```python
from build123d import *

# Parameters (mm, degrees)
SKETCH2_R          = 0.5
CUT_EXTRUDE1_DEPTH = 9.746515042
SKETCH3_R          = 33.25
SKETCH3_R_2        = 28.75
CUT_EXTRUDE3_DEPTH = 7.5


with BuildPart() as part:
    # Sketch1 → Revolve1 (revolve)
    with BuildSketch(Plane(origin=(0, 0, 0), x_dir=(1, 0, 0), z_dir=(0, 1, 0))):
        with BuildLine():
            Line((0, 2.406901823), (-37, 2.406901823))
            Line((-37, 2.406901823), (-37, -0.593098177))
            ThreePointArc((-37, -0.593098177), (-18.857679345, -5.739925328), (0, -5.593098177))
            Line((0, -5.593098177), (0, 2.406901823))
        make_face()
    revolve(axis=Axis((0, 0, -18.524642857), (0, 0, 1)))

    # Sketch2 → Cut-Extrude1 (cut, through all)
    with BuildSketch(Plane(origin=(0, 0, -2.406901823), x_dir=(-1, 0, 0), z_dir=(0, 0, -1))):
        Circle(SKETCH2_R)
    extrude(amount=-CUT_EXTRUDE1_DEPTH, mode=Mode.SUBTRACT)

    # Sketch3 → Cut-Extrude3 (cut)
    with BuildSketch(Plane.XY.offset(8)):
        Circle(SKETCH3_R)
        Circle(SKETCH3_R_2, mode=Mode.SUBTRACT)
    extrude(amount=-CUT_EXTRUDE3_DEPTH, mode=Mode.SUBTRACT)


solid = part.part
```
Can you work these out from the model? Positions are in its coordinate system, mm. Coordinates: 2 decimals unless noted, no trailing zeros. Answer as CSV lines item,"result". Start each with the question number.
1) For pin 1 (5 mm diameter, centred on y = 7.5, z = 0.5, fed in from -X); pin 2 (2 mm diameter, centred on x = -0.5, z = 2.5, fed in from -Y); pin 3 (1.5 mm diameter, centred on y = 24.5, z = 3.5, fed in from +X), each with a flat end and sliding along its axis, tell me the tip position at first contact or that it passes through.
2) Thinking about a two-plate mould opening in Y: for faces 1 (the flat face through (-1, -1, -2.407)), 2 (the cylindrical face through (-6.232, -28.066, 2.086)), 3 (the cylindrical face through (8.02, 36.12, -0.89)), which applies, pulls with the +Y half, pulls with the -Y half, needs draft (parallel to the pull), parting line crosses it, or undercut?
3) I need wall thicknesses on line 1 (X direction, y = 0, z = 1.25); line 2 (Y direction, x = 0, z = 2.25); line 3 (Y direction, x = 0, z = 1.3). Which ranges of each line are inside material? Lowest first, please. Write a range as from..to.
Check result:
1,pin 1,"stops at x = -36.66"
1,pin 2,"stops at y = -34.86"
1,pin 3,"stops at x = 16.2"
2,face 1,"needs draft"
2,face 2,"undercut"
2,face 3,"parting line crosses it"
3,line 1,"x = -35.47..-33.25, -28.75..-0.5, 0.5..28.75, 33.25..35.47"
3,line 2,"y = -28.75..-0.5, 0.5..28.75"
3,line 3,"y = -35.35..-33.25, -28.75..-0.5, 0.5..28.75, 33.25..35.35"
